Check sheet for the modelled part. Datum: model origin and axes. Units: mm. Face numbers are marked on the shaded views. A direction names the side the tool comes from. Round coordinates to 2 decimals unless told otherwise and drop trailing zeros. Order: outer loops, then holes, each group sorted by start corner. A loop starts at its lowest first (then second) coordinate and runs counter-clockwise, first axis right, second up. Notation, with made-up numbers: M -38,78.5 L -19,78.5 A17 cw -19,82.5 Z; hole C 2,-1.75 d1. An arc over 180 degrees is marked long. One line per item, written item: value. Start each with the question number.
(1) Cross-section at C-C, the plane x = 24.5. Enter the section's corners in (y, z).
(2) Access from +Z, -Z, +X, -X, +Y, -Y to the whole of each face (thin tool, end or side, straight path). Record for the marked faces 4 and 5.
(3) Cross-section at B-B, the plane x = 10.5. Enter the section's corners in (y, z).
(4) Thickness scan on L1, parallel to Y at x = 28.5, z = 4.25; L2, parallel to Y at x = 37, z = 0.25; L3, parallel to Z at x = 18, y = 9. Record the ranges inside material, lowest first.
(5) Release check for a two-part mould opening along Y. For the marked faces 1, 2 and 3 record: released by +Y, released by -Y, zero draft, split by the parting line, or undercut.
(6) Depth check by flat-ended pin: pin 1 Ø7.5 at (x, y) = (25.5, 3.5) entering from +Z; pin 2 Ø2 at (y, z) = (3.5, 1.5) entering from -X; pin 3 Ø3 at (y, z) = (0, 1.5) entering from +X. Enter the tip coordinate at first touch or a pass-through.
(7) Cross-section at A-A, the plane z = 2.5. Enter the section's corners in (x, y) (1 decimal).
Autodesk Inventor part; units mm, degrees
ref_plane "YZ Plane" through (0, 0, 0) normal (1, 0, 0) x (0, 1, 0)
ref_plane "XZ Plane" through (0, 0, 0) normal (0, 1, 0) x (-1, 0, 0)
ref_plane "XY Plane" through (0, 0, 0) normal (0, 0, 1) x (1, 0, 0)
sketch "Эскиз1" plane through (0, 0, 0) normal (0, 0, 1) x (1, 0, 0)
  arc A0 (37.9034, -0.2173) -> (42.261, 4.1403) centre (37.9034, 4.1403) ccw
  arc A1 (42.261, 8.15) -> (38.0283, 12.3827) centre (38.0283, 8.15) ccw
  arc A2 (43.261, 7.6552) -> (37.7725, 13.3827) centre (37.5283, 7.6552) ccw
  arc A3 (37.765, -1.2173) -> (43.261, 4.5105) centre (37.5283, 4.5105) ccw
  line L0 (37.765, -1.2173) -> (6.1001, -1.2173)
  line L1 (5.7034, -0.2173) -> (37.9034, -0.2173)
  line L2 (5.8283, 12.3827) -> (5.7034, -0.2173) construction
  arc A4 (5.8283, 12.3827) -> (5.7034, -0.2173) centre (6.0021, 6.0803) ccw
  arc A5 (6.1001, 13.3827) -> (6.1001, -1.2173) centre (6.1001, 6.0827) ccw
  line L3 (5.8283, 12.3827) -> (38.0283, 12.3827)
  line L4 (5.8283, 12.3827) -> (18.4289, 12.3827) construction
  line L5 (37.7725, 13.3827) -> (6.1001, 13.3827)
  line L6 (42.261, 8.15) -> (42.261, 4.1403)
  line L7 (43.261, 7.6552) -> (43.261, 4.5105)
  point P0 (0, 0)
  point P1 (0, 0)
  point P2 (0, 0)
  dimension "d10" = 1.5
  dimension "d0" = 90.568
  dimension "d1" = 4.2327
  dimension "d2" = 5.7327
  dimension "d3" = 5.7327
  dimension "d4" = 1
  dimension "d5" = 1
  dimension "d6" = 12.6
  dimension "d7" = 32.2
  dimension "d8" = 32.2
  dimension "d9" = 1
extrude "main_walls" add sketch "Эскиз1" along normal blind 2
sketch "Эскиз2" plane through (0, 0, 0) normal (0, 0, -1) x (-1, 0, 0)
  line L0 (-6.1001, 13.3827) -> (-37.7725, 13.3827)
  arc A0 (-37.7725, 13.3827) -> (-43.261, 7.6552) centre (-37.5283, 7.6552) ccw
  line L1 (-43.261, 7.6552) -> (-43.261, 4.5105)
  arc A1 (-43.261, 4.5105) -> (-37.765, -1.2173) centre (-37.5283, 4.5105) ccw
  line L2 (-37.765, -1.2173) -> (-6.1001, -1.2173)
  arc A2 (-6.1001, -1.2173) -> (-6.1001, 13.3827) centre (-6.1001, 6.0827) ccw
  point P0 (0, 0)
extrude "top" add sketch "Эскиз2" along normal blind 0.8
sketch "Эскиз3" plane through (0, 0, -0.8) normal (0, 0, -1) x (-1, 0, 0)
  line L0 (-6.1001, 13.3827) -> (-37.7725, 13.3827)
  arc A0 (-37.7725, 13.3827) -> (-43.261, 7.6552) centre (-37.5283, 7.6552) ccw
  line L1 (-43.261, 7.6552) -> (-43.261, 4.5105)
  arc A1 (-43.261, 4.5105) -> (-37.765, -1.2173) centre (-37.5283, 4.5105) ccw
  line L2 (-37.765, -1.2173) -> (-6.1001, -1.2173)
  arc A2 (-6.1001, -1.2173) -> (-6.1001, 13.3827) centre (-6.1001, 6.0827) ccw
  line L3 (1.1999, -1.8994) -> (1.1999, 13.1826)
  line L4 (-7.4001, 0.4827) -> (-12.1001, 0.4827)
  line L5 (-12.1001, 0.4827) -> (-12.1001, 6.1827)
  line L6 (-12.1001, 6.1827) -> (-7.4001, 6.1827)
  line L7 (-7.4001, 6.1827) -> (-7.4001, 0.4827)
  circle A3 centre (-4.6001, 5.0827) radius 1
  circle A4 centre (-5.4001, 9.3827) radius 0.6
  line L8 (-33.761, 4.8827) -> (-35.261, 4.8827)
  line L9 (-35.261, 4.8827) -> (-35.261, 6.8827)
  line L10 (-35.261, 6.8827) -> (-33.761, 6.8827)
  line L11 (-33.761, 6.8827) -> (-33.761, 4.8827)
  point P0 (0, 0)
  dimension "d15" = 4.7
  dimension "d16" = 5.7
  dimension "d17" = 1.7
  dimension "d18" = 2
  dimension "d19" = 1.2
  dimension "d20" = 5.8
  dimension "d21" = 2.8
  dimension "d22" = 6.3
  dimension "d23" = 4
  dimension "d24" = 0.8
  dimension "d25" = 1.5
  dimension "d26" = 2
  dimension "d27" = 6.1
  dimension "d28" = 8
extrude "Выдавливание5" cut sketch "Эскиз3" against normal blind 1.8 contours L4 L5 L6 L7 | A3 | A4 | L8 L9 L10 L11
sketch "Эскиз8" plane through (0, 0, -0.8) normal (0, 0, -1) x (-1, 0, 0)
  line L0 (-33.761, 6.8827) -> (-33.761, 4.8827)
  line L1 (-33.761, 4.8827) -> (-35.261, 4.8827)
  line L2 (-35.261, 4.8827) -> (-35.261, 6.8827)
  line L3 (-35.261, 6.8827) -> (-33.761, 6.8827)
  circle A0 centre (-4.6001, 5.0827) radius 1
  circle A1 centre (-5.4001, 9.3827) radius 0.6
  line L4 (-7.4001, 6.1827) -> (-7.4001, 0.4827)
  line L5 (-7.4001, 0.4827) -> (-12.1001, 0.4827)
  line L6 (-12.1001, 0.4827) -> (-12.1001, 6.1827)
  line L7 (-12.1001, 6.1827) -> (-7.4001, 6.1827)
  line L8 (-6.1001, 13.3827) -> (-37.7725, 13.3827)
  arc A2 (-37.7725, 13.3827) -> (-43.261, 7.6552) centre (-37.5283, 7.6552) ccw
  line L9 (-43.261, 7.6552) -> (-43.261, 4.5105)
  arc A3 (-43.261, 4.5105) -> (-37.765, -1.2173) centre (-37.5283, 4.5105) ccw
  line L10 (-37.765, -1.2173) -> (-6.1001, -1.2173)
  arc A4 (-6.1001, -1.2173) -> (-6.1001, 13.3827) centre (-6.1001, 6.0827) ccw
  arc A5 (-6.1001, -1.8173) -> (-6.1001, 13.9827) centre (-6.1001, 6.0827) ccw
  line L11 (-6.1001, 13.9827) -> (-37.7813, 13.9827)
  line L12 (-6.1001, -1.8173) -> (-37.7733, -1.8173)
  arc A6 (-43.8609, 4.5105) -> (-37.7733, -1.8173) centre (-37.5283, 4.5105) ccw
  arc A7 (-37.7813, 13.9827) -> (-43.8609, 7.6552) centre (-37.5283, 7.6552) ccw
  line L13 (-43.8609, 7.6552) -> (-43.8609, 4.5105)
  point P0 (0, 0)
  dimension "d73" = 7.3
  dimension "d74" = 7.9
extrude "Выдавливание8" add sketch "Эскиз8" against normal blind 8 contours L12 A6 L13 A7 L11 A5
fillet "Сопряжение3" radius 1 6 edges at (-1.7999, 6.0827, -0.8) (21.9407, 13.9827, -0.8) (21.9367, -1.8173, -0.8) (42.0919, 0.1202, -0.8) (42.0947, 12.0426, -0.8) (43.8609, 6.0828, -0.8)
equation "\"d2\" = d1 + d10"
equation "\"d3\" = d1 + d10"
equation "\"d5\" = d4"
equation "\"d7\" = d8"
equation "\"d9\" = d4"
properties part number "top"
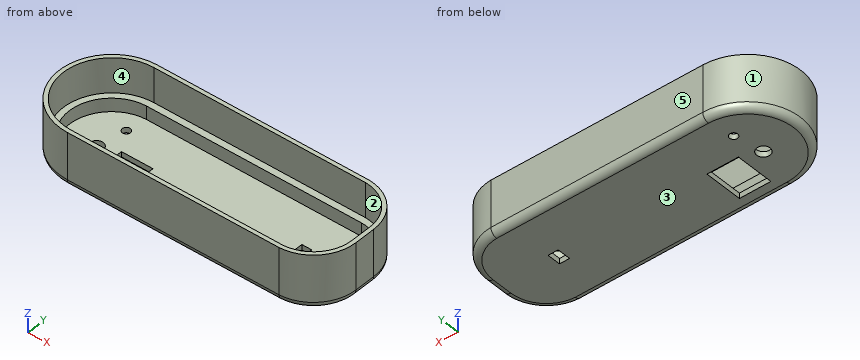
Values found:
1. outline: M -1.82,0.2 A1 ccw -0.82,-0.8 L 12.98,-0.8 A1 ccw 13.98,0.2 L 13.98,7.2 L 13.38,7.2 L 13.38,2 L 12.38,2 L 12.38,0 L -0.22,0 L -0.22,2 L -1.22,2 L -1.22,7.2 L -1.82,7.2 Z
2. face 4: +Z
2. face 5: +Z, -Z, +X, -X, +Y
3. outline: M -1.82,0.2 A1 ccw -0.82,-0.8 L 0.48,-0.8 L 0.48,0 L -0.22,0 L -0.22,2 L -1.22,2 L -1.22,7.2 L -1.82,7.2 Z; M 6.18,-0.8 L 12.98,-0.8 A1 ccw 13.98,0.2 L 13.98,7.2 L 13.38,7.2 L 13.38,2 L 12.38,2 L 12.38,0 L 6.18,0 Z
4. L1: -1.82 to -1.22, 13.38 to 13.98
4. L2: -1.82 to -0.22, 12.38 to 13.98
4. L3: -0.8 to 0
5. face 1: split by the parting line
5. face 2: undercut
5. face 3: zero draft
6. pin 1: z = 2
6. pin 2: x = -1.64
6. pin 3: x = 43.1
7. outline: M 6.1,-1.8 L 37.8,-1.8 A6.3 ccw 43.9,4.5 L 43.9,7.7 A6.3 ccw 37.8,14 L 6.1,14 A7.9 ccw Z; hole M 6.1,-1.2 L 37.8,-1.2 A5.7 ccw 43.3,4.5 L 43.3,7.7 A5.7 ccw 37.8,13.4 L 6.1,13.4 A7.3 ccw Z
